```python
from build123d import *

# Parameters (mm, degrees)
BOSS_EXTRUDE1_DEPTH = 5.5372
SKETCH3_R           = 2.0955
CUT_EXTRUDE1_DEPTH  = 361.538157474


with BuildPart() as part:
    # Sketch2 → Boss-Extrude1 (new body)
    with BuildSketch(Plane.XY):
        with BuildLine():
            Line((300.094596165, 188.940880076), (299.62806999, 188.353043175))
            ThreePointArc((299.62806999, 188.353043175), (299.150949063, 188.019920142), (298.569281031, 188.003257744))
            ThreePointArc((298.569281031, 188.003257744), (298.073872939, 188.308521819), (297.827235612, 188.835575292))
            Line((297.827235612, 188.835575292), (297.717130543, 189.577920069))
            ThreePointArc((297.717130543, 189.577920069), (296.712124973, 190.444856977), (295.707119404, 189.577920069))
            Line((295.707119404, 189.577920069), (295.597014335, 188.835575292))
            ThreePointArc((295.597014335, 188.835575292), (295.350377008, 188.308521819), (294.854968915, 188.003257744))
            ThreePointArc((294.854968915, 188.003257744), (294.273300884, 188.019920142), (293.796179957, 188.353043175))
            Line((293.796179957, 188.353043175), (293.329653782, 188.940880076))
            ThreePointArc((293.329653782, 188.940880076), (292.025824973, 189.189166677), (291.588933073, 187.935874506))
            Line((291.588933073, 187.935874506), (291.864751675, 187.237932536))
            ThreePointArc((291.864751675, 187.237932536), (291.914684221, 186.658172176), (291.638280265, 186.146101686))
            ThreePointArc((291.638280265, 186.146101686), (291.126209774, 185.86969773), (290.546449415, 185.919630276))
            Line((290.546449415, 185.919630276), (289.848507445, 186.195448877))
            ThreePointArc((289.848507445, 186.195448877), (288.595215274, 185.758556977), (288.843501875, 184.454728169))
            Line((288.843501875, 184.454728169), (289.431338776, 183.988201994))
            ThreePointArc((289.431338776, 183.988201994), (289.764461809, 183.511081067), (289.781124207, 182.929413036))
            ThreePointArc((289.781124207, 182.929413036), (289.475860132, 182.434004943), (288.948806659, 182.187367616))
            Line((288.948806659, 182.187367616), (288.206461882, 182.077262547))
            ThreePointArc((288.206461882, 182.077262547), (287.339524973, 181.072256977), (288.206461882, 180.067251408))
            Line((288.206461882, 180.067251408), (288.948806659, 179.957146339))
            ThreePointArc((288.948806659, 179.957146339), (289.475860132, 179.710509012), (289.781124207, 179.215100919))
            ThreePointArc((289.781124207, 179.215100919), (289.764461809, 178.633432888), (289.431338776, 178.156311961))
            Line((289.431338776, 178.156311961), (288.843501875, 177.689785786))
            ThreePointArc((288.843501875, 177.689785786), (288.595215274, 176.385956977), (289.848507445, 175.949065077))
            Line((289.848507445, 175.949065077), (290.546449415, 176.224883679))
            ThreePointArc((290.546449415, 176.224883679), (291.126209774, 176.274816225), (291.638280265, 175.998412269))
            ThreePointArc((291.638280265, 175.998412269), (291.914684221, 175.486341779), (291.864751675, 174.906581419))
            Line((291.864751675, 174.906581419), (291.588933073, 174.208639449))
            ThreePointArc((291.588933073, 174.208639449), (292.025824973, 172.955347278), (293.329653782, 173.203633879))
            Line((293.329653782, 173.203633879), (293.796179957, 173.79147078))
            ThreePointArc((293.796179957, 173.79147078), (294.273300884, 174.124593813), (294.854968915, 174.141256211))
            ThreePointArc((294.854968915, 174.141256211), (295.350377008, 173.835992136), (295.597014335, 173.308938663))
            Line((295.597014335, 173.308938663), (295.707119404, 172.566593886))
            ThreePointArc((295.707119404, 172.566593886), (296.712124973, 171.699656977), (297.717130543, 172.566593886))
            Line((297.717130543, 172.566593886), (297.827235612, 173.308938663))
            ThreePointArc((297.827235612, 173.308938663), (298.073872939, 173.835992136), (298.569281031, 174.141256211))
            ThreePointArc((298.569281031, 174.141256211), (299.150949063, 174.124593813), (299.62806999, 173.79147078))
            Line((299.62806999, 173.79147078), (300.094596165, 173.203633879))
            ThreePointArc((300.094596165, 173.203633879), (301.398424973, 172.955347278), (301.835316873, 174.208639449))
            Line((301.835316873, 174.208639449), (301.559498271, 174.906581419))
            ThreePointArc((301.559498271, 174.906581419), (301.509565726, 175.486341779), (301.785969682, 175.998412269))
            ThreePointArc((301.785969682, 175.998412269), (302.298040172, 176.274816225), (302.877800532, 176.224883679))
            Line((302.877800532, 176.224883679), (303.575742502, 175.949065077))
            ThreePointArc((303.575742502, 175.949065077), (304.829034673, 176.385956977), (304.580748071, 177.689785786))
            Line((304.580748071, 177.689785786), (303.99291117, 178.156311961))
            ThreePointArc((303.99291117, 178.156311961), (303.659788137, 178.633432888), (303.64312574, 179.215100919))
            ThreePointArc((303.64312574, 179.215100919), (303.948389815, 179.710509012), (304.475443288, 179.957146339))
            Line((304.475443288, 179.957146339), (305.217788065, 180.067251408))
            ThreePointArc((305.217788065, 180.067251408), (306.084724973, 181.072256977), (305.217788065, 182.077262547))
            Line((305.217788065, 182.077262547), (304.475443288, 182.187367616))
            ThreePointArc((304.475443288, 182.187367616), (303.948389815, 182.434004943), (303.64312574, 182.929413036))
            ThreePointArc((303.64312574, 182.929413036), (303.659788137, 183.511081067), (303.99291117, 183.988201994))
            Line((303.99291117, 183.988201994), (304.580748071, 184.454728169))
            ThreePointArc((304.580748071, 184.454728169), (304.829034673, 185.758556977), (303.575742502, 186.195448877))
            Line((303.575742502, 186.195448877), (302.877800532, 185.919630276))
            ThreePointArc((302.877800532, 185.919630276), (302.298040172, 185.86969773), (301.785969682, 186.146101686))
            ThreePointArc((301.785969682, 186.146101686), (301.509565726, 186.658172176), (301.559498271, 187.237932536))
            Line((301.559498271, 187.237932536), (301.835316873, 187.935874506))
            ThreePointArc((301.835316873, 187.935874506), (301.398424973, 189.189166677), (300.094596165, 188.940880076))
        make_face()
    extrude(amount=BOSS_EXTRUDE1_DEPTH)

    # Sketch3 → Cut-Extrude1 (cut, through all)
    with BuildSketch(Plane.XY.offset(5.5372)):
        with Locations((296.712124973, 181.072256977)):
            Circle(SKETCH3_R)
    extrude(amount=-CUT_EXTRUDE1_DEPTH, mode=Mode.SUBTRACT)


solid = part.part
```
Check sheet for the modelled part. Datum: model origin and axes. Units: mm. Give positions to 0.01 mm unless a question says otherwise; leave off trailing zeros. Loops run counter-clockwise (first coordinate to the right, second up) from the corner with the lowest first, then second, coordinate; pieces in that order, holes last. Notation, with made-up numbers: (-15.5, 36.25) - (-5.5, 36.25) arc R13 cw to (-5.5, 41.25) - close; hole circle Ø3 at (67.25, 47). An arc over 180 degrees is marked (long way). One line per question, with ' | ' between items. Start each with the question number.
1. Cross-section at B-B, the plane y = 180.5. Enter the section's corners in (x, z), plus the area to 3 significant figures.
2. Cross-section at A-A, the plane x = 296.25. Enter the section's corners in (y, z).
3. Cross-section at C-C, the plane y = 175.25. Enter the section's corners in (x, z).
4. Gauge pin test, flat ends, axial feed: pin 1 Ø1 at (x, z) = (289.5, 3.5) entering from +Y; pin 2 Ø3 at (x, z) = (302.5, 2.5) entering from +Y; pin 3 Ø2 at (y, z) = (174, 0.5) entering from +X. Record the tip position at first contact, or that the pin passes through.
5. Draft check along Y on faces 1 (the cylindrical face through (296.7, 171.7, 2.7)), 2 (the cylindrical face through (298.65, 180.27, 2.81)), 3 (the flat face through (294, 181, 0)). Enter one of: released by +Y, released by -Y, zero draft, split by the parting line, or undercut.
6. Material ranges on line 1 along X through (y, z) = (174, 5); line 2 along Y through (x, z) = (304.25, 5.25); line 3 along X through (y, z) = (173, 3.15), recorded low to high. Write a range as [from, to].
7. Cross-section at D-D, the plane x = 303.25. Enter the section's corners in (y, z).
Check result:
1) outline: (287.52, 0) - (294.7, 0) - (294.7, 5.54) - (287.52, 5.54) - close; (298.73, 0) - (305.91, 0) - (305.91, 5.54) - (298.73, 5.54) - close | area: 79.5 mm2
2) outline: (171.81, 0) - (179.03, 0) - (179.03, 5.54) - (171.81, 5.54) - close; (183.12, 0) - (190.33, 0) - (190.33, 5.54) - (183.12, 5.54) - close
3) outline: (291.94, 0) - (301.49, 0) - (301.49, 5.54) - (291.94, 5.54) - close
4) pin 1: stops at y = 186.27 | pin 2: stops at y = 189.32 | pin 3: stops at x = 301.91
5) face 1: released by -Y | face 2: undercut | face 3: zero draft
6) line 1: x = [291.53, 294.02], [295.16, 298.26], [299.4, 301.89] | line 2: y = [175.92, 177.95], [179.9, 182.25], [184.19, 186.22] | line 3: x = [291.96, 293.11], [295.64, 297.78], [300.31, 301.47]
7) outline: (176.08, 0) - (186.07, 0) - (186.07, 5.54) - (176.08, 5.54) - close
